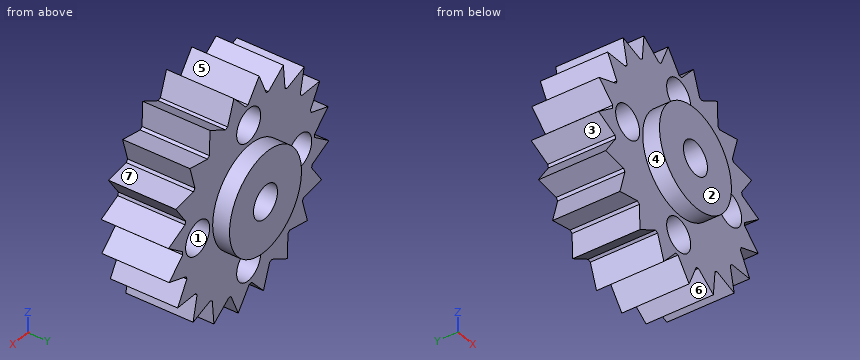
```python
from build123d import *

# Parameters (mm, degrees)
F0_R      = 8.73125
F1_DEPTH  = 3.175
F2_R      = 4.7625
F3_DEPTH  = 1.5875
F4_R      = 1.5875
F5_DEPTH  = 7.9385
F6_R      = 1.5875
F7_DEPTH  = 6.351
F10_DEPTH = 6.35
F11_COUNT = 20


with BuildPart() as f1:
    # F0 (on Front) → F1 (new body, symmetric)
    with BuildSketch(Plane.XZ):
        Circle(F0_R)
    extrude(amount=F1_DEPTH, both=True)

    # F2 (on face) → F3 (join)
    with BuildSketch(Plane.XZ.offset(3.175)):
        Circle(F2_R)
    extrude(amount=F3_DEPTH)

    # F4 (on face) → F5 (cut, through all)
    with BuildSketch(Plane.XZ.offset(4.7625)):
        Circle(F4_R)
    extrude(amount=-F5_DEPTH, mode=Mode.SUBTRACT)

    # F6 (on face) → F7 (cut, through all)
    with BuildSketch(Plane.XZ.offset(3.175)):
        with Locations((0, 6.7137391306)):
            Circle(F6_R)
        with Locations((0, -6.7137391306)):
            Circle(F6_R)
        with Locations((-6.750960571, 0)):
            Circle(F6_R)
        with Locations((6.750960571, 0)):
            Circle(F6_R)
    extrude(amount=-F7_DEPTH, mode=Mode.SUBTRACT)

    # F8: F1 across plane


with BuildPart() as f1_1:
    add(f1.part)
    add(f1.part.mirror(Plane.XZ))



with BuildPart() as f10:
    # F9 (on face) → F10 (new body, through all)
    with BuildSketch(Plane.XZ.offset(3.175)):
        with BuildLine():
            Line((-1.3848210597, 10.604101041), (-2.324559949, 8.4161242627))
            ThreePointArc((-2.324559949, 8.4161242627), (-1.1306393797, 8.6577353364), (0.0852877991, 8.7308334398))
            Line((0.0852877991, 8.7308334398), (-1.3848210597, 10.604101041))
        make_face()
    extrude(amount=-F10_DEPTH)


with BuildPart() as f1_2:
    add(f1_1.part)

    add(f10.part)  # F11 merges F10
    # F11: F10 ×20 about axis
    f11_axis = Axis((0, -3.175, 0), (0, -1, 0))
    for i in range(1, F11_COUNT):
        add(f10.part.rotate(f11_axis, i * 360 / F11_COUNT))


solid = f1_2.part
```
The model under review builds one solid part; all positions refer to its coordinate system, in mm. Face numbers are marked on the shaded views. A direction names the side the tool comes from. Round coordinates to 2 decimals unless told otherwise and drop trailing zeros. Loops run counter-clockwise (first coordinate to the right, second up) from the corner with the lowest first, then second, coordinate; pieces in that order, holes last.
Item 1: Take a section at B-B (x = -1). Write out the cut boundary in (y, z) (1 decimal), then the cut area to 3 significant figures.
Determined:
outline: (-4.8, -4.7) - (-3.2, -4.7) - (-3.2, -5.5) - (3.2, -5.5) - (3.2, -4.7) - (4.8, -4.7) - (4.8, -1.2) - (-4.8, -1.2) - close; (-4.8, 1.2) - (4.8, 1.2) - (4.8, 4.7) - (3.2, 4.7) - (3.2, 5.5) - (-3.2, 5.5) - (-3.2, 4.7) - (-4.8, 4.7) - close; (-3.2, -9.4) - (3.2, -9.4) - (3.2, -7.9) - (-3.2, -7.9) - close; (-3.2, 7.9) - (3.2, 7.9) - (3.2, 10.1) - (-3.2, 10.1) - close
area: 98.8 mm2
Item 2: Take a section at C-C (y = 4). Write out the cut boundary in (x, z) (1 decimal).
Determined:
outline: circle Ø9.5 at (0, 0); hole circle Ø3.2 at (0, 0)
Item 3: For line 1 (X direction, y = -2.25, z = 9.5); line 2 (X direction, y = -1.5, z = 1.25); line 3 (Z direction, x = 9, y = 1), list the stretches that pass through material, from the lowest coordinate up.
Determined:
line 1: x = -4.61 to -4.36, -1.86 to -0.52, 1.07 to 2.33
line 2: x = -9.7 to -7.73, -5.77 to -0.98, 0.98 to 5.77, 7.73 to 10.43
line 3: z = -5.13 to -4.45, -2.51 to -0.63, 0.13 to 2.07, 3.62 to 4.65
Item 4: For the marked faces 4, 5, 6 and 7, list the 3-axis set-ups (+Z, -Z, +X, -X, +Y, -Y) from which the entire face can be reached by the end or side of a thin tool; tool diameter is ignored.
Determined:
face 4: -Y
face 5: +Z, +Y, -Y
face 6: -Z, +Y, -Y
face 7: +X, +Y, -Y
Item 5: Take a section at D-D (x = -4.25). Write out the cut boundary in (y, z) (1 decimal).
Determined:
outline: (-4.8, -2.1) - (-3.2, -2.1) - (-3.2, -8.9) - (3.2, -8.9) - (3.2, -2.1) - (4.8, -2.1) - (4.8, 2.1) - (3.2, 2.1) - (3.2, 9.4) - (-3.2, 9.4) - (-3.2, 2.1) - (-4.8, 2.1) - close
Item 6: Clearance check with flat-ended pins moving along their axes: pin 1 Ø2.5 at (x, z) = (0, 6.71) entering from -Y; pin 2 Ø1 at (x, z) = (-6, 5) entering from -Y (3 decimals); pin 3 Ø2 at (x, y) = (5.5, 0) entering from -Z; pin 4 Ø1.5 at (x, y) = (-6.5, -2) entering from -Z. State where each tip first meets the part, or that it passes through.
Determined:
pin 1: passes through
pin 2: stops at y = -3.175
pin 3: stops at z = -9.66
pin 4: stops at z = -7.24
Item 7: Mouldability with a two-part tool opening along X and no side actions: class the marked faces 1, 2 and 3 as released by +X, released by -X, zero draft, split by the parting line, or undercut.
Determined:
face 1: undercut
face 2: zero draft
face 3: released by -X
Item 8: Take a section at A-A (z = 5.75). Write out the cut boundary in (x, y) (1 decimal), then the cut area to 3 significant figures.
Determined:
outline: (-6.9, -3.2) - (-1.3, -3.2) - (-1.3, 3.2) - (-6.9, 3.2) - close; (1.3, -3.2) - (7.3, -3.2) - (7.3, 3.2) - (1.3, 3.2) - close
area: 74.2 mm2
